Verification items for this drawing (mm, ordinates from the low corner). A direction names the side the tool comes from. Round coordinates to 2 decimals unless told otherwise and drop trailing zeros. Order: outer loops, then holes, each group sorted by start corner. A loop starts at its lowest first (then second) coordinate and runs counter-clockwise, first axis right, second up.
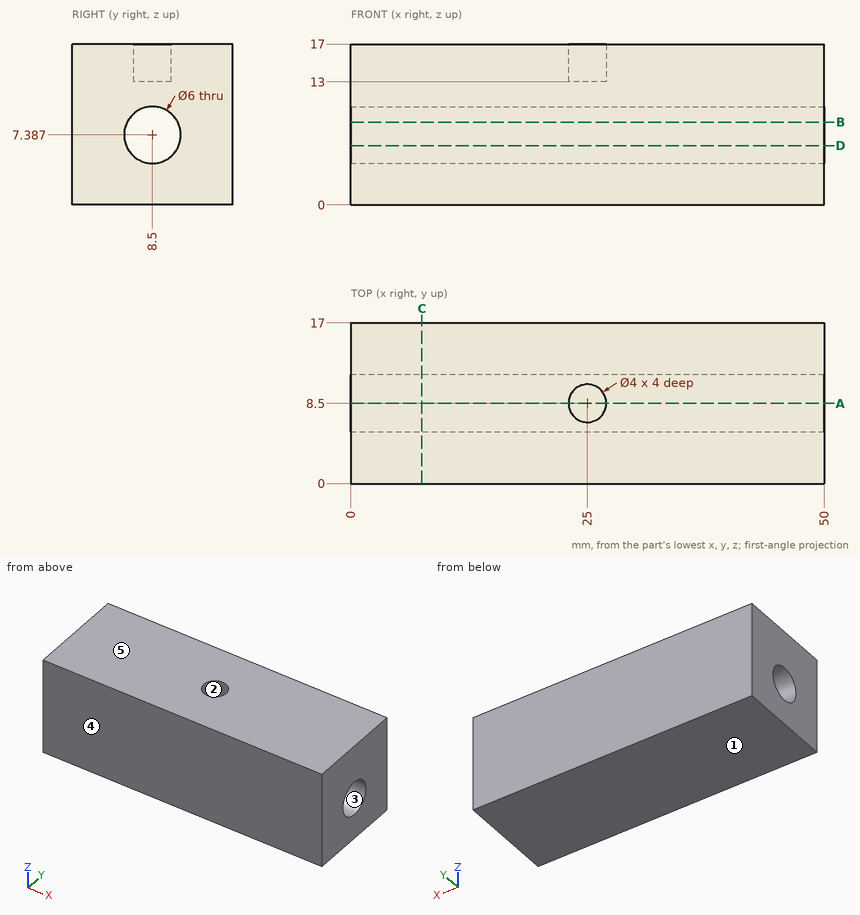
Item 1: Sectioned sample at B-B (z = 8.75). Record the cut outline in (x, y).
Answer:
outline: (0, 0) - (50, 0) - (50, 5.83) - (0, 5.83) - close; (0, 11.17) - (50, 11.17) - (50, 17) - (0, 17) - close
Item 2: Sectioned sample at D-D (z = 6.25). Record the cut outline in (x, y).
Answer:
outline: (0, 0) - (50, 0) - (50, 5.72) - (0, 5.72) - close; (0, 11.28) - (50, 11.28) - (50, 17) - (0, 17) - close
Item 3: Access from +Z, -Z, +X, -X, +Y, -Y to the whole of each face (thin tool, end or side, straight path). Record for the marked faces 1 and 2.
Answer:
face 1: -Z, +X, -X, +Y, -Y
face 2: +Z
Item 4: Sectioned sample at A-A (y = 8.5). Record the cut outline in (x, z).
Answer:
outline: (0, 0) - (50, 0) - (50, 4.39) - (0, 4.39) - close; (0, 10.39) - (50, 10.39) - (50, 17) - (27, 17) - (27, 13) - (23, 13) - (23, 17) - (0, 17) - close
Item 5: Release check for a two-part mould opening along Z. For the marked faces 3, 4 and 5 record: released by +Z, released by -Z, zero draft, split by the parting line, or undercut.
Answer:
face 3: undercut
face 4: zero draft
face 5: released by +Z
Item 6: Sectioned sample at C-C (x = 7.5). Record the cut outline in (y, z).
Answer:
outline: (0, 0) - (17, 0) - (17, 17) - (0, 17) - close; hole circle Ø6 at (8.5, 7.39)
Item 7: Scan lines: line 1 along Z through (x, y) = (18, 8.5); line 2 along Y through (x, z) = (38.5, 9); line 3 along Y through (x, z) = (18, 6.25) (1 decimal). Record each from-to range of solid material in increasing order.
Answer:
line 1: z = 0 to 4.39, 10.39 to 17
line 2: y = 0 to 5.97, 11.03 to 17
line 3: y = 0 to 5.7, 11.3 to 17
